Here's how the part is built. I have some questions about the finished solid (model axes, mm). A direction names the side the tool comes from. Round coordinates to 2 decimals unless told otherwise and drop trailing zeros. Order: outer loops, then holes, each group sorted by start corner. A loop starts at its lowest first (then second) coordinate and runs counter-clockwise, first axis right, second up. Notation, with made-up numbers: (73.5, 50.25) - (114.5, 50.25) arc R32 ccw to (114.5, 78.25) - close; hole circle Ø4 at (87.25, -36). An arc over 180 degrees is marked (long way). Answer as a JSON object with one key per item and string values.
```python
from build123d import *

# Parameters (mm, degrees)
SKETCH1_R                      = 25
SKETCH1_R_2                    = 4
BOSS_EXTRUDE1_DEPTH            = 5
SKETCH2_R                      = 5.15
CUT_EXTRUDE1_DEPTH             = 3
SKETCH3_R                      = 11.125
CUT_EXTRUDE2_DEPTH             = 2
SKETCH4_R                      = 1.25
CUT_EXTRUDE3_DEPTH             = 4
M4_CLEARANCE_HOLE1_D           = 4.5
M4_CLEARANCE_HOLE1_DEPTH       = 7.6
M4_CLEARANCE_HOLE1_CSINK_D     = 4.55
M4_CLEARANCE_HOLE1_CSINK_ANGLE = 90
M4_CLEARANCE_HOLE1_TIP         = 1.351936393


with BuildPart() as part:
    # Sketch1 → Boss-Extrude1 (new body)
    with BuildSketch(Plane(origin=(0, 0, 0), x_dir=(0, 0, -1), z_dir=(1, 0, 0))):
        Circle(SKETCH1_R)
        Circle(SKETCH1_R_2, mode=Mode.SUBTRACT)
    extrude(amount=BOSS_EXTRUDE1_DEPTH)

    # Sketch2 → Cut-Extrude1 (cut)
    with BuildSketch(Plane(origin=(5, 0, 0), x_dir=(0, 0, -1), z_dir=(1, 0, 0))):
        Circle(SKETCH2_R)
    extrude(amount=-CUT_EXTRUDE1_DEPTH, mode=Mode.SUBTRACT)

    # Sketch3 → Cut-Extrude2 (cut)
    with BuildSketch(Plane(origin=(5, 0, 0), x_dir=(0, 0, -1), z_dir=(1, 0, 0))):
        Circle(SKETCH3_R)
    extrude(amount=-CUT_EXTRUDE2_DEPTH, mode=Mode.SUBTRACT)

    # Sketch4 → Cut-Extrude3 (cut, through all)
    with BuildSketch(Plane(origin=(3, 0, 0), x_dir=(0, 0, -1), z_dir=(1, 0, 0))):
        with Locations((0, 7)):
            Circle(SKETCH4_R)
        with Locations((6.062177826, -3.5)):
            Circle(SKETCH4_R)
        with Locations((-6.062177826, -3.5)):
            Circle(SKETCH4_R)
    extrude(amount=-CUT_EXTRUDE3_DEPTH, mode=Mode.SUBTRACT)

    # M4 Clearance Hole1
    with Locations(Plane(origin=(5, 0, 0), x_dir=(0, 0, -1), z_dir=(1, 0, 0))):
        with Locations((0, 21.213203436), (21.213203436, 0), (-21.213203436, 0), (0, -21.213203436)):
            CounterSinkHole(M4_CLEARANCE_HOLE1_D / 2, M4_CLEARANCE_HOLE1_CSINK_D / 2, depth=M4_CLEARANCE_HOLE1_DEPTH, counter_sink_angle=M4_CLEARANCE_HOLE1_CSINK_ANGLE)
            with Locations((0, 0, -(M4_CLEARANCE_HOLE1_DEPTH + M4_CLEARANCE_HOLE1_TIP / 2))):  # 118° drill point
                Cone(0, M4_CLEARANCE_HOLE1_D / 2, M4_CLEARANCE_HOLE1_TIP, mode=Mode.SUBTRACT)


solid = part.part
```
1. If I drill on L1, parallel to Y at x = 2.3, z = 0; L2, parallel to Y at x = 3.15, z = 0 (3 decimals); L3, parallel to Y at x = 1, z = -1, over which ranges is the centre line in solid material (lowest first)? Write a range as [from, to].
Responses:
{"L1": "[-25, -23.46], [-18.96, -5.15], [5.15, 5.75], [8.25, 18.96], [23.46, 25]", "L2": "[-25, -23.463], [-18.963, -11.125], [11.125, 18.963], [23.463, 25]", "L3": "[-24.98, -23.23], [-19.2, -3.87], [3.87, 6.25], [7.75, 19.2], [23.23, 24.98]"}
2. For faces 4 (the face through (2.453, 19.017, -0.488)), 5 (the face through (4.01, 7.52, 8.2)), which set-ups out of +Z, -Z, +X, -X, +Y, -Y let a thin tool reach every point of the face, with its end or its side?
Responses:
{"face 4": "+X, -X", "face 5": "+X"}
3. For P1, Ø1.5, axis at x = 1, y = -15.5, coming from the +Z side; P2, Ø4, axis at y = 0, z = -21.21, coming from the -X side; P3, Ø2, axis at x = 0.5, y = 6, coming from the +Z side; P4, Ø6.5, axis at y = -1.5, z = 5.5, coming from the +X side, each with a flat end and sliding along its axis, tell me the tip position at first contact or that it passes through.
Responses:
{"P1": "z = 20.19", "P2": "through", "P3": "z = 24.49", "P4": "x = 3"}
4. Imagine slicing it at C-C (y = 7). List the corners of the cut face in (x, z) for me.
Responses:
{"outline": "(0, -24) - (5, -24) - (5, -8.65) - (3, -8.65) - (3, -1.25) - (0, -1.25) - close; (0, 1.25) - (3, 1.25) - (3, 8.65) - (5, 8.65) - (5, 24) - (0, 24) - close"}
5. Imagine slicing it at A-A (y = 0). List the corners of the cut face in (x, z) for me (3 decimals), plus the area to 3 significant figures.
Responses:
{"outline": "(0, -25) - (5, -25) - (5, -23.488) - (4.975, -23.463) - (0, -23.463) - close; (0, -18.963) - (4.975, -18.963) - (5, -18.938) - (5, -11.125) - (3, -11.125) - (3, -5.15) - (2, -5.15) - (2, -4) - (0, -4) - close; (0, 4) - (2, 4) - (2, 5.15) - (3, 5.15) - (3, 11.125) - (5, 11.125) - (5, 18.938) - (4.975, 18.963) - (0, 18.963) - close; (0, 23.463) - (4.975, 23.463) - (5, 23.488) - (5, 25) - (0, 25) - close", "area": "134 mm2"}
6. Imagine slicing it at D-D (x = 4.4). List the corners of the cut face in (y, z) for me (3 decimals), plus the area to 3 significant figures.
Responses:
{"outline": "circle Ø50 at (0, 0); hole circle Ø4.5 at (-21.213, 0); hole circle Ø22.25 at (0, 0); hole circle Ø4.5 at (0, -21.213); hole circle Ø4.5 at (0, 21.213); hole circle Ø4.5 at (21.213, 0)", "area": "1,510 mm2"}
7. Thinking about a two-plate mould opening in Y: for faces 1 (the face through (2, -3, -3)), 2 (the face through (0, -5, 0)), 3 (the face through (2.465, 7.509, -23.846)), which applies, pulls with the +Y half, pulls with the -Y half, needs draft (parallel to the pull), parting line crosses it, or undercut?
Responses:
{"face 1": "undercut", "face 2": "needs draft", "face 3": "parting line crosses it"}
8. Imagine slicing it at B-B (z = 6). List the corners of the cut face in (x, y) for me, plus the area to 3 significant figures.
Responses:
{"outline": "(0, -24.27) - (5, -24.27) - (5, -9.37) - (3, -9.37) - (3, -4.75) - (0, -4.75) - close; (0, -2.25) - (3, -2.25) - (3, 9.37) - (5, 9.37) - (5, 24.27) - (0, 24.27) - close", "area": "198 mm2"}
